The drawing under review shows one solid part. Ordinate dimensions are in mm from its lowest x, y, z. Give positions to 0.01 mm unless a question says otherwise; leave off trailing zeros. Loops run counter-clockwise (first coordinate to the right, second up) from the corner with the lowest first, then second, coordinate; pieces in that order, holes last. Notation, with made-up numbers: (56, 38.5) - (63, 38.5) arc R29 cw to (63, 71.5) - close; hole circle Ø8 at (28.25, 70). An arc over 180 degrees is marked (long way). Write each question's results on one line, items separated by ' | '.
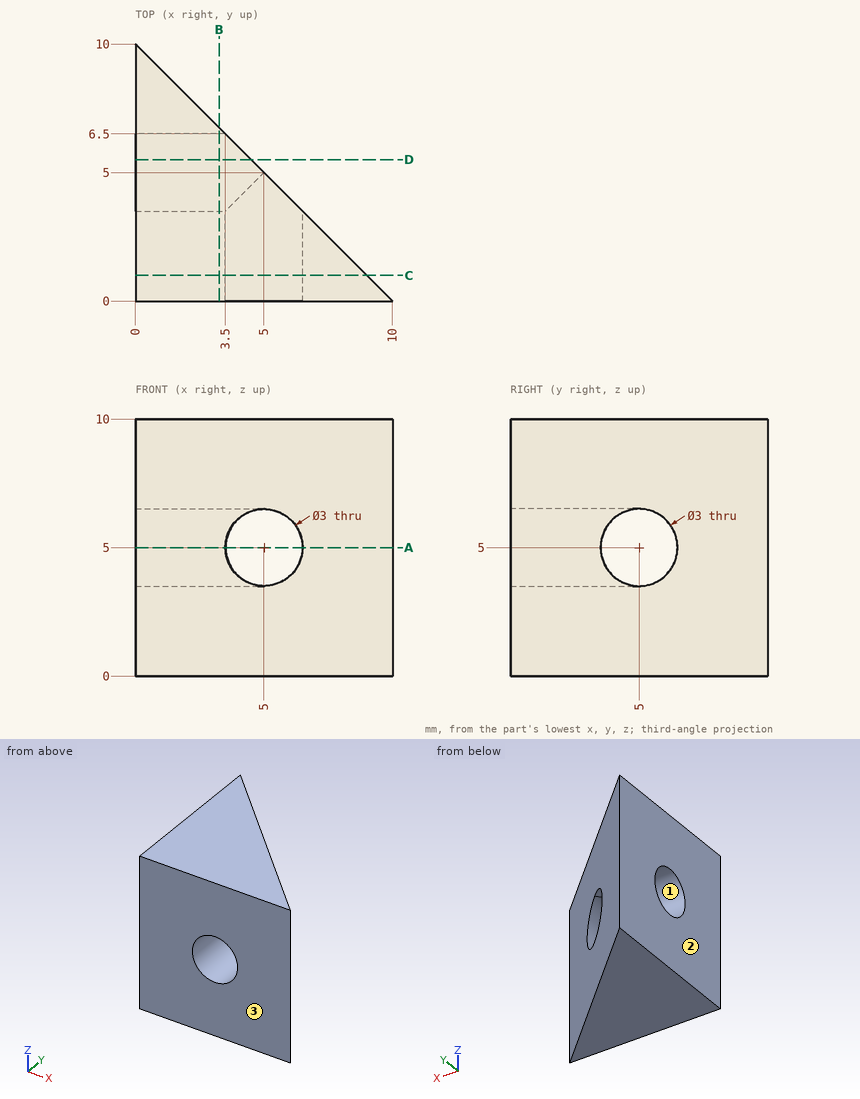
(1) Draft analysis for pull direction Y (two halves, no side actions). For the marked faces 1, 2 and 3, state which applies: pulls with the +Y half, pulls with the -Y half, needs draft (parallel to the pull), parting line crosses it, or undercut.
Answers below:
face 1: undercut | face 2: needs draft | face 3: pulls with the -Y half
(2) Take a section at A-A on z = 5. Give the boundary of the cut face in (x, y).
Answers below:
outline: (0, 0) - (3.5, 0) - (3.5, 3.5) - (0, 3.5) - close; (0, 6.5) - (3.5, 6.5) - (0, 10) - close; (6.5, 0) - (10, 0) - (6.5, 3.5) - close
(3) Take a section at C-C on y = 1. Give the boundary of the cut face in (x, z), plus the area to 3 significant figures.
Answers below:
outline: (0, 0) - (9, 0) - (9, 10) - (0, 10) - close; hole circle Ø3 at (5, 5) | area: 82.9 mm2
(4) Take a section at D-D on y = 5.5. Give the boundary of the cut face in (x, z), plus the area to 3 significant figures.
Answers below:
outline: (0, 0) - (4.5, 0) - (4.5, 3.59) - (0, 3.59) - close; (0, 6.41) - (4.5, 6.41) - (4.5, 10) - (0, 10) - close | area: 32.3 mm2
(5) Take a section at B-B on x = 3.25. Give the boundary of the cut face in (y, z).
Answers below:
outline: (0, 0) - (6.75, 0) - (6.75, 10) - (0, 10) - close; hole circle Ø3 at (5, 5)
(6) Insertion check: P1, Ø1.5, axis at x = 2.5, z = 2, coming from the +Y side; P2, Ø5, axis at x = 5, z = 5, coming from the +Y side; P3, Ø3, axis at y = 4, z = 6, coming from the +X side. Each pin has a flat end and moves straight along its axis. Give the tip position at first contact, or say it passes through.
Answers below:
P1: y = 8.25 | P2: y = 7.5 | P3: x = 7.5
(7) Wall thickness on line 1 along Z through (x, y) = (3.25, 5); line 2 along Y through (x, z) = (0.75, 5.25); line 3 along X through (y, z) = (5, 8.75): over which ranges is each line inside the solid? List them lowest first. Write a range as from..to.
Answers below:
line 1: 0..3.5, 6.5..10 | line 2: 0..3.52, 6.48..9.25 | line 3: 0..5
